```python
from build123d import *

# Parameters (mm, degrees)
SKETCH1_W           = 55
SKETCH1_H           = 10
BOSS_EXTRUDE1_DEPTH = 1
SKETCH2_W           = 7
SKETCH2_H           = 10
BOSS_EXTRUDE2_DEPTH = 23.9
CUT_EXTRUDE2_REACH  = 63.196
SKETCH4_R           = 1
SKETCH5_W           = 55
SKETCH5_H           = 10
BOSS_EXTRUDE3_DEPTH = 9
SKETCH6_W           = 55
SKETCH6_H           = 10
BOSS_EXTRUDE4_DEPTH = 10


with BuildPart() as part:
    # Sketch1 → Boss-Extrude1 (new body)
    with BuildSketch(Plane(origin=(0, 0, 0), x_dir=(1, 0, 0), z_dir=(0, 1, 0))):
        with Locations((27.5, 5)):
            Rectangle(SKETCH1_W, SKETCH1_H)
    extrude(amount=BOSS_EXTRUDE1_DEPTH)

    # Sketch2 → Boss-Extrude2 (add)
    with BuildSketch(Plane(origin=(0, 1, 0), x_dir=(1, 0, 0), z_dir=(0, 1, 0))):
        with Locations((51.5, 5)):
            Rectangle(SKETCH2_W, SKETCH2_H)
        with Locations((3.5, 5)):
            Rectangle(SKETCH2_W, SKETCH2_H)
    extrude(amount=BOSS_EXTRUDE2_DEPTH)

    # Sketch4 → Cut-Extrude2 (cut, up to next)
    with BuildSketch(Plane.XY, mode=Mode.PRIVATE) as cut_extrude2_sk1:
        with Locations((2.5, 17.95)):
            Circle(SKETCH4_R)
    cut_extrude2_tool1 = extrude(cut_extrude2_sk1.sketch, amount=-CUT_EXTRUDE2_REACH, mode=Mode.PRIVATE) & part.part
    # Sketch4 → Cut-Extrude2 (cut, up to next)
    with BuildSketch(Plane.XY, mode=Mode.PRIVATE) as cut_extrude2_sk2:
        with Locations((2.5, 8.35)):
            Circle(SKETCH4_R)
    cut_extrude2_tool2 = extrude(cut_extrude2_sk2.sketch, amount=-CUT_EXTRUDE2_REACH, mode=Mode.PRIVATE) & part.part
    # Sketch4 → Cut-Extrude2 (cut, up to next)
    with BuildSketch(Plane.XY, mode=Mode.PRIVATE) as cut_extrude2_sk3:
        with Locations((52.5, 8.35)):
            Circle(SKETCH4_R)
    cut_extrude2_tool3 = extrude(cut_extrude2_sk3.sketch, amount=-CUT_EXTRUDE2_REACH, mode=Mode.PRIVATE) & part.part
    # Sketch4 → Cut-Extrude2 (cut, up to next)
    with BuildSketch(Plane.XY, mode=Mode.PRIVATE) as cut_extrude2_sk4:
        with Locations((52.5, 17.95)):
            Circle(SKETCH4_R)
    cut_extrude2_tool4 = extrude(cut_extrude2_sk4.sketch, amount=-CUT_EXTRUDE2_REACH, mode=Mode.PRIVATE) & part.part
    add(cut_extrude2_tool1.solids().sort_by_distance((2.5, 17.95, 0))[0], mode=Mode.SUBTRACT)
    add(cut_extrude2_tool2.solids().sort_by_distance((2.5, 8.35, 0))[0], mode=Mode.SUBTRACT)
    add(cut_extrude2_tool3.solids().sort_by_distance((52.5, 8.35, 0))[0], mode=Mode.SUBTRACT)
    add(cut_extrude2_tool4.solids().sort_by_distance((52.5, 17.95, 0))[0], mode=Mode.SUBTRACT)

    # Sketch5 → Boss-Extrude3 (add)
    with BuildSketch(Plane.XZ):
        with Locations((27.5, -5)):
            Rectangle(SKETCH5_W, SKETCH5_H)
    extrude(amount=BOSS_EXTRUDE3_DEPTH)

    # Sketch6 → Boss-Extrude4 (add)
    with BuildSketch(Plane(origin=(0, 24.9, 0), x_dir=(1, 0, 0), z_dir=(0, 1, 0))):
        with Locations((27.5, 5)):
            Rectangle(SKETCH6_W, SKETCH6_H)
    extrude(amount=BOSS_EXTRUDE4_DEPTH)


solid = part.part
```
Verification items for the finished model (mm, model axes). A direction names the side the tool comes from. Coordinates: 2 decimals unless noted, no trailing zeros. Loops run counter-clockwise (first coordinate to the right, second up) from the corner with the lowest first, then second, coordinate; pieces in that order, holes last. Notation, with made-up numbers: (-16.75, 71) - (2.25, 71) arc R21 ccw to (2.25, 107) - close; hole circle Ø6 at (59, 78). An arc over 180 degrees is marked (long way). Put each result on its own line as item: value.
Item 1: Section check C-C (z = -8.5). Enter the section's corners in (x, y), then the cut area to 3 significant figures.
Conclusion:
outline: (0, -9) - (55, -9) - (55, 34.9) - (0, 34.9) - close; hole circle Ø2 at (2.5, 8.35); hole circle Ø2 at (2.5, 17.95); hole (7, 1) - (48, 1) - (48, 24.9) - (7, 24.9) - close; hole circle Ø2 at (52.5, 8.35); hole circle Ø2 at (52.5, 17.95)
area: 1,420 mm2
Item 2: Scan lines: line 1 along Y through (x, z) = (52.5, -2.75); line 2 along Y through (x, z) = (36.5, -1.75); line 3 along X through (y, z) = (11.5, -6). Record each from-to range of solid material in increasing order.
Conclusion:
line 1: y = -9 to 7.35, 9.35 to 16.95, 18.95 to 34.9
line 2: y = -9 to 1, 24.9 to 34.9
line 3: x = 0 to 7, 48 to 55
Item 3: Draft check along Y on faces 1 (the face through (52.96, 17.06, -4.93)), 2 (the face through (27, -9, -5)), 3 (the face through (27, -2, -10)). Enter one of: pulls with the +Y half, pulls with the -Y half, needs draft (parallel to the pull), parting line crosses it, or undercut.
Conclusion:
face 1: undercut
face 2: pulls with the -Y half
face 3: needs draft
Item 4: Section check D-D (x = 18.5). Enter the section's corners in (y, z).
Conclusion:
outline: (-9, -10) - (1, -10) - (1, 0) - (-9, 0) - close; (24.9, -10) - (34.9, -10) - (34.9, 0) - (24.9, 0) - close
Item 5: Set-up check for faces 4 (the face through (27, -2, 0)), 5 (the face through (27, 24.9, -5)): record each of +Z, -Z, +X, -X, +Y, -Y from which the full face is reachable in a straight line by a thin tool's end or side.
Conclusion:
face 4: +Z, +X, -X, +Y, -Y
face 5: +Z, -Z
Item 6: Section check B-B (y = 8.35). Enter the section's corners in (x, z), then the cut area to 3 significant figures.
Conclusion:
outline: (0, -10) - (1.5, -10) - (1.5, 0) - (0, 0) - close; (3.5, -10) - (7, -10) - (7, 0) - (3.5, 0) - close; (48, -10) - (51.5, -10) - (51.5, 0) - (48, 0) - close; (53.5, -10) - (55, -10) - (55, 0) - (53.5, 0) - close
area: 100 mm2
Item 7: Section check A-A (x = 2.5). Enter the section's corners in (y, z), then the cut area to 3 significant figures.
Conclusion:
outline: (-9, -10) - (7.35, -10) - (7.35, 0) - (-9, 0) - close; (9.35, -10) - (16.95, -10) - (16.95, 0) - (9.35, 0) - close; (18.95, -10) - (34.9, -10) - (34.9, 0) - (18.95, 0) - close
area: 399 mm2
Item 8: Gauge pin test, flat end, axial feed: pin 1 Ø1.5 at (y, z) = (14.5, -1.5) entering from -X. Record the tip position at first contact, or that the pin passes through.
Conclusion:
pin 1: stops at x = 0
